Check sheet for the modelled part. Datum: model origin and axes. Units: mm. A direction names the side the tool comes from. Round coordinates to 2 decimals unless told otherwise and drop trailing zeros. Write each loop counter-clockwise with the first axis right and the second up, starting at its lowest first coordinate (ties: lowest second). Pieces come first, ordered by that corner, then holes. Notation, with made-up numbers: M 5.5,48 L 59.5,48 A19 cw 59.5,66 Z; hole C -39,43.25 d11. An arc over 180 degrees is marked long. Answer in a Markdown table with one row per item.
```python
from build123d import *

# Parameters (mm, degrees)
BOSS_EXTRUDE1_DEPTH = 3
CUT_EXTRUDE1_START  = -1.25
CUT_EXTRUDE1_DEPTH  = 1.25
FILLET2_R           = 10
CHAMFER1_SIZE       = 5
CHAMFER1_SIZE_2     = 1.339745962
FILLET3_START       = 7.722693831
FILLET3_DEPTH       = 14.027306169
FILLET3_2_ANGLE     = 41.120463
FILLET3_3_ANGLE     = 41.120463
FILLET4_R           = 0.5
SKETCH10_R          = 1.4
CUT_EXTRUDE3_DEPTH  = 10


with BuildPart() as part:
    # Sketch1 → Boss-Extrude1 (new body)
    with BuildSketch(Plane(origin=(0, 0, 0), x_dir=(1, 0, 0), z_dir=(0, 1, 0))):
        with BuildLine():
            Line((-3.15, -4.2), (-3.15, -21.75))
            Line((-3.15, -21.75), (3.15, -21.75))
            Line((3.15, -21.75), (3.15, -4.2))
            ThreePointArc((3.15, -4.2), (0, 5.25), (-3.15, -4.2))
        make_face()
    extrude(amount=BOSS_EXTRUDE1_DEPTH)

    # Sketch2 → Cut-Extrude1 (cut)
    with BuildSketch(Plane(origin=(0, 3, 0), x_dir=(1, 0, 0), z_dir=(0, 1, 0)).offset(CUT_EXTRUDE1_START)):
        with BuildLine():
            Line((-3.15, -4.2), (-3.15, -5.25))
            Line((-3.15, -5.25), (3.15, -5.25))
            Line((3.15, -5.25), (3.15, -4.2))
            ThreePointArc((3.15, -4.2), (0, 5.25), (-3.15, -4.2))
        make_face()
    extrude(amount=CUT_EXTRUDE1_DEPTH, mode=Mode.SUBTRACT)

    # Cut-Sweep1: sweep along a path in Sketch9
    with BuildLine(Plane(origin=(0, 0, 0), x_dir=(1, 0, 0), z_dir=(0, 1, 0))) as cut_sweep1_path:
        CenterArc((0, 0), 3.5, 0, 360)
    # Sketch8 → Cut-Sweep1 (sweep, cut)
    with BuildSketch(Plane(origin=(0, 0, 0), x_dir=(0, 0, -1), z_dir=(1, 0, 0))):
        with BuildLine():
            Line((0, 3.5), (0, 0))
            Line((0, 0), (3.5, 0))
            ThreePointArc((3.5, 0), (2.474873734, 2.474873734), (0, 3.5))
        make_face()
    sweep(path=cut_sweep1_path.line, mode=Mode.SUBTRACT)

    # Fillet2
    # the kernel refuses this fillet: 10 mm, written as the material it adds along each edge
    with BuildSketch(Plane(origin=(-3.15, 0, 4.2), x_dir=(0, 0, 1), z_dir=(0, 1, 0))) as fillet2_piece_1_section:
        with BuildLine():
            CenterArc((3.522693831, -10), FILLET2_R, 90, 30.424740483)
            ThreePointArc((-1.541367698, -1.37704918), (-0.702247096, -0.765127664), (0, 0))
            Line((0, 0), (3.522693831, 0))
        make_face()
    fillet2_piece_1 = extrude(amount=1.75, mode=Mode.PRIVATE)
    fillet2_piece_1 = split(fillet2_piece_1, bisect_by=Plane(origin=(-3.15, 0, 5.25), z_dir=(0, 0, 1)), keep=Keep.TOP, mode=Mode.PRIVATE)
    add(fillet2_piece_1)
    with BuildSketch(Plane(origin=(-3.15, 0, 4.2), x_dir=(0, 0, 1), z_dir=(0, 1, 0))) as fillet2_piece_2_section:
        with BuildLine():
            CenterArc((3.522693831, -10), FILLET2_R, 90, 30.424740483)
            ThreePointArc((-1.541367698, -1.37704918), (-0.702247096, -0.765127664), (0, 0))
            Line((0, 0), (3.522693831, 0))
        make_face()
    fillet2_piece_2 = extrude(amount=1.75, mode=Mode.PRIVATE)
    fillet2_piece_2 = split(fillet2_piece_2, bisect_by=Plane(origin=(-3.15, 0, 5.25), z_dir=(0, 0, -1)), keep=Keep.TOP, mode=Mode.PRIVATE)
    add(fillet2_piece_2)
    with BuildSketch(Plane(origin=(-3.15, 0, 4.2), x_dir=(0, 0, 1), z_dir=(0, 1, 0))) as fillet2_piece_3_section:
        with BuildLine():
            CenterArc((3.522693831, -10), FILLET2_R, 90, 30.424740483)
            ThreePointArc((-1.541367698, -1.37704918), (-0.702247096, -0.765127664), (0, 0))
            Line((0, 0), (3.522693831, 0))
        make_face()
    fillet2_piece_3 = extrude(amount=10.556734576, mode=Mode.PRIVATE)
    fillet2_piece_3 = split(fillet2_piece_3, bisect_by=Plane(origin=(-3.15, 3, 4.2), z_dir=(0, -1, 0)), keep=Keep.TOP, mode=Mode.PRIVATE)
    fillet2_piece_3 = split(fillet2_piece_3, bisect_by=Plane(origin=(-3.15, 0, 5.25), z_dir=(0, 0, 1)), keep=Keep.TOP, mode=Mode.PRIVATE)
    fillet2_piece_3 = split(fillet2_piece_3, bisect_by=Plane(origin=(-3.15, 1.75, 4.2), z_dir=(0, 1, 0)), keep=Keep.TOP, mode=Mode.PRIVATE)
    add(fillet2_piece_3)
    with BuildSketch(Plane(origin=(3.15, 0, 4.2), x_dir=(0.6662386483372984, 0, -0.7457386026361313), z_dir=(0, 1, 0))) as fillet2_piece_4_section:
        with BuildLine():
            CenterArc((4.035377709, -9.804340803), FILLET2_R, 101.352680936, 30.424740483)
            Line((-2.627008775, -2.346954776), (0, 0))
            ThreePointArc((0, 0), (1.033450389, -0.102721079), (2.066900778, 0))
        make_face()
    fillet2_piece_4 = extrude(amount=1.75, mode=Mode.PRIVATE)
    fillet2_piece_4 = split(fillet2_piece_4, bisect_by=Plane(origin=(3.15, 0, 5.25), z_dir=(0, 0, -1)), keep=Keep.TOP, mode=Mode.PRIVATE)
    add(fillet2_piece_4)
    with BuildSketch(Plane(origin=(3.15, 0, 4.2), x_dir=(0.6662386483372984, 0, -0.7457386026361313), z_dir=(0, 1, 0))) as fillet2_piece_5_section:
        with BuildLine():
            CenterArc((4.035377709, -9.804340803), FILLET2_R, 101.352680936, 30.424740483)
            Line((-2.627008775, -2.346954776), (0, 0))
            ThreePointArc((0, 0), (1.033450389, -0.102721079), (2.066900778, 0))
        make_face()
    fillet2_piece_5 = extrude(amount=1.75, mode=Mode.PRIVATE)
    fillet2_piece_5 = split(fillet2_piece_5, bisect_by=Plane(origin=(3.15, 0, 5.25), z_dir=(0, 0, 1)), keep=Keep.TOP, mode=Mode.PRIVATE)
    add(fillet2_piece_5)
    with BuildSketch(Plane(origin=(3.15, 0, 4.2), x_dir=(0.6662386483372984, 0, -0.7457386026361313), z_dir=(0, 1, 0))) as fillet2_piece_6_section:
        with BuildLine():
            CenterArc((4.035377709, -9.804340803), FILLET2_R, 101.352680936, 30.424740483)
            Line((-2.627008775, -2.346954776), (0, 0))
            ThreePointArc((0, 0), (1.033450389, -0.102721079), (2.066900778, 0))
        make_face()
    fillet2_piece_6 = extrude(amount=10.556734576, mode=Mode.PRIVATE)
    fillet2_piece_6 = split(fillet2_piece_6, bisect_by=Plane(origin=(3.15, 3, 4.2), z_dir=(0, -1, 0)), keep=Keep.TOP, mode=Mode.PRIVATE)
    fillet2_piece_6 = split(fillet2_piece_6, bisect_by=Plane(origin=(3.15, 0, 5.25), z_dir=(0, 0, 1)), keep=Keep.TOP, mode=Mode.PRIVATE)
    fillet2_piece_6 = split(fillet2_piece_6, bisect_by=Plane(origin=(3.15, 1.75, 4.2), z_dir=(0, 1, 0)), keep=Keep.TOP, mode=Mode.PRIVATE)
    add(fillet2_piece_6)

    # Chamfer1
    # the kernel refuses this chamfer: 5, 1.339745962 mm, written as the material it takes off along each edge
    with BuildSketch(Plane(origin=(16.444140104, 3, 5.25), x_dir=(0, 0, 1), z_dir=(-1, 0, 0))) as chamfer1_piece_1_section:
        Polygon((CHAMFER1_SIZE, 0), (0, -CHAMFER1_SIZE_2), (0, 0), align=None)
    chamfer1_piece_1 = extrude(amount=32.888280208, mode=Mode.PRIVATE)
    chamfer1_piece_1 = split(chamfer1_piece_1, bisect_by=Plane(origin=(16.444140104, 1.75, 5.25), z_dir=(0, 1, 0)), keep=Keep.TOP, mode=Mode.PRIVATE)
    add(chamfer1_piece_1, mode=Mode.SUBTRACT)

    # Fillet3: read off the stored shape, not the designer's step
    # Fillet3 outline → Fillet3 (cut)
    with BuildSketch(Plane.XY.offset(FILLET3_START)):
        with BuildLine():
            ThreePointArc((-3.15, 0), (-2.271320344, 2.121320344), (-0.15, 3))
            Line((-0.15, 3), (-3.15, 3))
            Line((-3.15, 3), (-3.15, 0))
        make_face()
        with BuildLine():
            Line((3.15, 0), (3.15, 3))
            Line((3.15, 3), (0.15, 3))
            ThreePointArc((0.15, 3), (2.271320344, 2.121320344), (3.15, 0))
        make_face()
    extrude(amount=FILLET3_DEPTH, mode=Mode.SUBTRACT)

    # Fillet3 2 outline → Fillet3 2 (revolve, cut)
    with BuildSketch(Plane(origin=(-13.15, 0, 7.722693831), x_dir=(1, 0, 0), z_dir=(0, 0, 1))):
        with BuildLine():
            ThreePointArc((10, 0), (10.289308449, 1.285360382), (11.101434209, 2.322810353))
            Line((11.101434209, 2.322810353), (10, 2.322810353))
            Line((10, 2.322810353), (10, 0))
        make_face()
    revolve(axis=Axis((-13.15, 0, 7.722693831), (0, 1, 0)), revolution_arc=FILLET3_2_ANGLE, mode=Mode.SUBTRACT)

    # Fillet3 3 outline → Fillet3 3 (revolve, cut)
    with BuildSketch(Plane(origin=(13.15, 0, 7.722693831), x_dir=(-0.7533285646584991, 0, -0.6576443367577688), z_dir=(0.6576443367577688, 0, -0.7533285646584991))):
        with BuildLine():
            ThreePointArc((10, 0), (10.289308449, 1.285360382), (11.101434209, 2.322810353))
            Line((11.101434209, 2.322810353), (10, 2.322810353))
            Line((10, 2.322810353), (10, 0))
        make_face()
    revolve(axis=Axis((13.15, 0, 7.722693831), (0, 1, 0)), revolution_arc=FILLET3_3_ANGLE, mode=Mode.SUBTRACT)

    # Fillet4
    fillet4_edges = [part.edges().sort_by_distance(p)[0] for p in [
        (-1e-09, 1.75, -5.25),
    ]]
    fillet(fillet4_edges, radius=FILLET4_R)

    # Mirror2: read off the stored shape, not the designer's step
    # Mirror2: part across plane


with BuildPart() as part_1:
    add(part.part)
    add(part.part.mirror(Plane.ZX))

    # Sketch10 → Cut-Extrude3 (cut)
    with BuildSketch(Plane.XY.offset(21.75)):
        Circle(SKETCH10_R)
    extrude(amount=-CUT_EXTRUDE3_DEPTH, mode=Mode.SUBTRACT)


solid = part_1.part
```
1. Section check B-B, the plane y = 0.25. Record the cut outline in (x, z).
Found:
| item | result |
|---|---|
| outline | M -4.66,2.42 A5.25 ccw long 4.66,2.42 A10.01 cw 3.14,7.72 L 3.14,21.75 L 1.38,21.75 L 1.38,11.75 L -1.38,11.75 L -1.38,21.75 L -3.14,21.75 L -3.14,7.72 A10.01 cw Z; hole C 0,0 d6.98 |
2. Section check A-A, the plane z = 0. Record the cut outline in (x, y).
Found:
| item | result |
|---|---|
| outline | M -5.25,-1.25 A0.5 ccw -4.75,-1.75 L -3.03,-1.75 A3.5 cw -3.03,1.75 L -4.75,1.75 A0.5 ccw -5.25,1.25 Z; M 3.03,-1.75 L 4.75,-1.75 A0.5 ccw 5.25,-1.25 L 5.25,1.25 A0.5 ccw 4.75,1.75 L 3.03,1.75 A3.5 cw Z |
3. Section check C-C, the plane z = 10. Record the cut outline in (x, y), and give its area (3 significant figures).
Found:
| item | result |
|---|---|
| outline | M -0.78,-2.93 L 0.78,-2.93 A3 ccw 0.78,2.93 L -0.78,2.93 A3 ccw Z |
| area | 29.9 mm2 |
4. Access from +Z, -Z, +X, -X, +Y, -Y to the whole of each face (thin tool, end or side, straight path). Record for faces 1 (the face through (1.4, 0.7, 21.75)), 2 (the face through (-3, -1.75, 2)), 3 (the face through (-1.4, 0.06, 16.82)), 4 (the face through (-3, 1.75, 2)).
Found:
| item | result |
|---|---|
| face 1 | +Z, +X, -X, +Y, -Y |
| face 2 | -Z, +X, -X, -Y |
| face 3 | +Z |
| face 4 | -Z, +X, -X, +Y |
5. Draft check along Y on faces 5 (the face through (0, 0, 11.75)), 6 (the face through (0.154, 0.018, -5.248)), 7 (the face through (0.039, 2.245, 7.432)). Enter one of: +Y half, -Y half, draft (parallel to the pull), parting line (faces both ways), or undercut.
Found:
| item | result |
|---|---|
| face 5 | undercut |
| face 6 | draft |
| face 7 | +Y half |
6. Go/stop test with flat-tipped pins: pin 1 (4.5 mm diameter, centred on x = -0.5, z = 1.5, fed in from -Y); pin 2 (1 mm diameter, centred on x = -2.5, z = 15.5, fed in from -Y); pin 3 (3 mm diameter, centred on x = 3.5, z = -1, fed in from +Y). Record where each tip stops, or that it passes through.
Found:
| item | result |
|---|---|
| pin 1 | stops at y = -1.75 |
| pin 2 | stops at y = -2.36 |
| pin 3 | stops at y = 1.75 |
7. Scan lines: L1, parallel to Y at x = 0, z = 19.5; L2, parallel to Z at x = 1.5, y = -0.5; L3, parallel to Y at x = 2, z = 3.75. Record each from-to range of solid material in increasing order.
Found:
| item | result |
|---|---|
| L1 | y = -3 to -1.4, 1.4 to 3 |
| L2 | z = -5.03 to -3.12, 3.12 to 21.75 |
| L3 | y = -1.75 to 1.75 |
